Verification items for this drawing (mm, ordinates from the low corner). A direction names the side the tool comes from. Round coordinates to 2 decimals unless told otherwise and drop trailing zeros. Order: outer loops, then holes, each group sorted by start corner. A loop starts at its lowest first (then second) coordinate and runs counter-clockwise, first axis right, second up. Notation, with made-up numbers: (49, 17.5) - (101, 17.5) arc R15 cw to (101, 44.5) - close; hole circle Ø5 at (77.25, -21). An arc over 180 degrees is marked (long way). Return JSON: item names as keys, results as strings. Group by question number.
Q1. Sectioned sample at D-D, the plane y = 4. Record the cut outline in (x, z), then the cut area to 3 significant figures.
Q2. Material ranges on line 1 along X through (y, z) = (28, 17.5); line 2 along Z through (x, y) = (42, 23); line 3 along Z through (x, y) = (28, 13), recorded low to high.
Q3. Sectioned sample at B-B, the plane z = 26.5. Record the cut outline in (x, y) (1 decimal).
Q4. Sectioned sample at A-A, the plane y = 39. Record the cut outline in (x, z), then the cut area to 3 significant figures.
Q5. Gauge pin test, flat ends, axial feed: pin 1 Ø4 at (x, y) = (9.5, 39.5) entering from +Z; pin 2 Ø12 at (x, y) = (20, 24.5) entering from +Z; pin 3 Ø5 at (x, y) = (19.5, 18) entering from +Z. Record the tip position at first contact, or that the pin passes through.
Q6. Sectioned sample at C-C, the plane x = 36. Record the cut outline in (y, z).
Q7. Draft check along X on the marked faces 5, 6, 7 and 8. Enter one of: pulls with the +X half, pulls with the -X half, needs draft (parallel to the pull), parting line crosses it, or undercut.
Q8. Tool access check on the marked faces 1, 2, 3 and 4. Record the directions out of +Z, -Z, +X, -X, +Y, -Y that give a thin tool (end or side, any length) a straight path to the whole face; none if there is none.
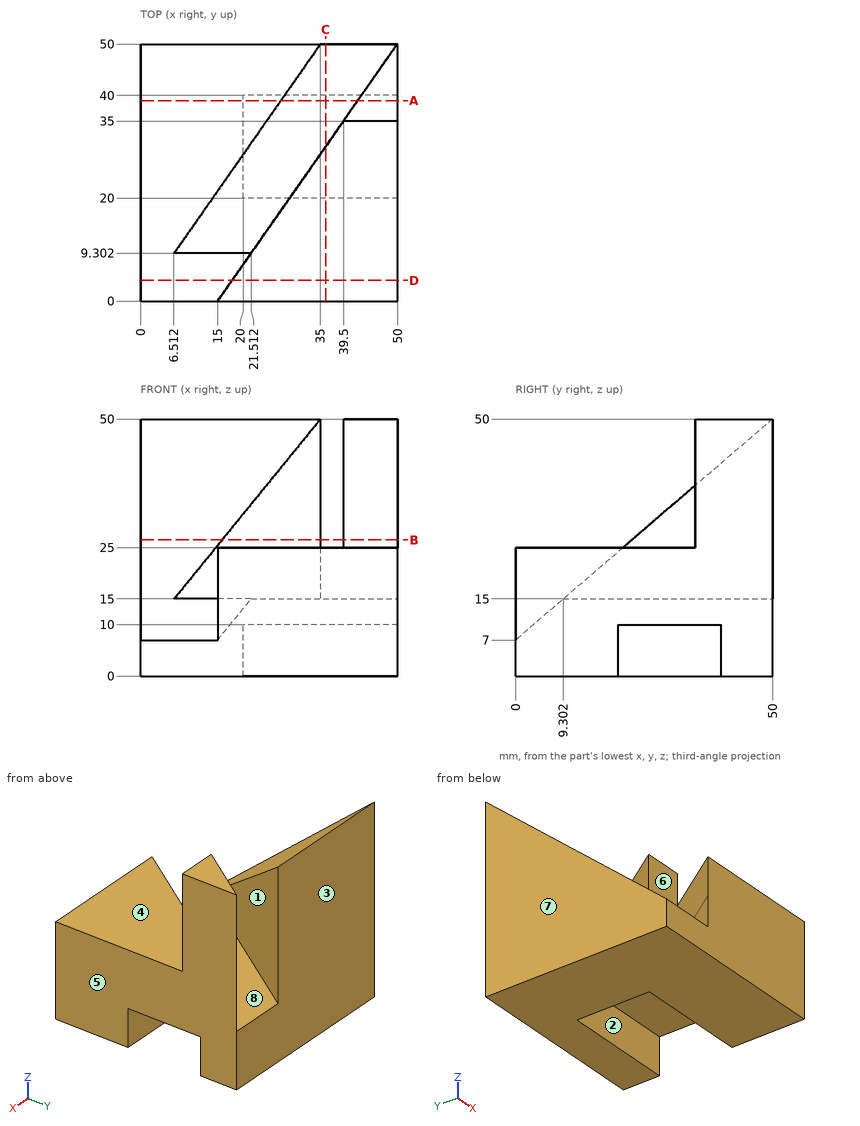
Reply:
{
 "1": {"outline": "(0, 0) - (50, 0) - (50, 25) - (17.8, 25) - (17.8, 10.44) - (0, 10.44) - close", "area": "991 mm^2"},
 "2": {"line 1": "0 to 19.6, 34.6 to 50", "line 2": "10 to 25", "line 3": "0 to 25"},
 "3": {"outline": "(0, 22.7) - (15.9, 22.7) - (35, 50) - (0, 50) - close; (39.5, 35) - (50, 35) - (50, 50) - close"},
 "4": {"outline": "(0, 0) - (20, 0) - (20, 10) - (50, 10) - (50, 50) - (42.3, 50) - (42.3, 15) - (27.3, 15) - (27.3, 40.54) - (0, 40.54) - close", "area": "1,420 mm^2"},
 "5": {"pin 1": "z = 42.69", "pin 2": "z = 33.23", "pin 3": "z = 15"},
 "6": {"outline": "(0, 0) - (20, 0) - (20, 10) - (40, 10) - (40, 0) - (50, 0) - (50, 15) - (30, 15) - (30, 25) - (0, 25) - close"},
 "7": {"face 5": "pulls with the +X half", "face 6": "needs draft", "face 7": "pulls with the -X half", "face 8": "undercut"},
 "8": {"face 1": "+Z", "face 2": "-Z, +X", "face 3": "+Z, -Z, +X, -X, +Y", "face 4": "+Z, +X, -Y"}
}
